Can you work these out from the model? Positions are in its coordinate system, mm. A direction names the side the tool comes from. Give positions to 0.01 mm unless a question says otherwise; leave off trailing zeros. Order: outer loops, then holes, each group sorted by start corner. A loop starts at its lowest first (then second) coordinate and runs counter-clockwise, first axis right, second up.
Item 1: If I drill on line 1 along Y through (x, z) = (-9.5, 10.5); line 2 along X through (y, z) = (38, 5); line 3 along Y through (x, z) = (14.5, -16.5), over which ranges is the centre line in solid material (lowest first)?
Item 2: I want a section at B-B, the plane y = 28.5. Write out the boundary of the cut face in (x, z).
Item 3: If we mould it in two halves opening along Z, with no side actions, what happens to faces 3 (the cylindrical face through (-10.14, 10.726, 12.559)), 4 (the cylindrical face through (-10.14, 17.16, -27.48)), 5 (the flat face through (-10, 20, -15))? For each: +Z half, -Z half, draft (parallel to the pull), parting line (faces both ways), or undercut.
Item 4: I want a section at C-C, the plane z = 22.5. Write out the boundary of the cut face in (x, y).
Item 5: I'm going to push flat-ended pins straight in: pin 1 Ø4 at (x, z) = (-5.5, 19) entering from +Y; pin 2 Ø10 at (x, z) = (5.5, -2) entering from +Y; pin 3 Ø8 at (x, z) = (0, -5.5) entering from +Y; pin 4 Ø3 at (x, z) = (-0.5, -3) entering from -Y. Where does each tip first touch, or does it pass through?
Item 6: Which directions (+Z, -Z, +X, -X, +Y, -Y) give clear straight access to the entire face, cutting with the end or side of a thin tool? Please do faces 1 (the flat face through (20, 5, 0)), 2 (the flat face through (10, 10, 0)).
Item 7: I want a section at D-D, the plane z = 5. Write out the boundary of the cut face in (x, y), then the cut area to 3 significant figures.
Item 8: I want a section at A-A, the plane x = -3.5. Write out the boundary of the cut face in (y, z), then the cut area to 3 significant figures.
```python
from build123d import *

# Parameters (mm, degrees)
SKETCH1_W              = 40
SKETCH1_H              = 61
BOSS_EXTRUDE1_DEPTH    = 40
SKETCH2_W              = 20
SKETCH2_H              = 61
CUT_EXTRUDE1_DEPTH     = 30
CUT_EXTRUDE3_START     = -20
CUT_EXTRUDE3_OUTLINE_R = 9.5
CUT_EXTRUDE3_DEPTH     = 20


# Read off the part's stored shape, not the designer's step: Cut-Extrude3
with BuildPart() as part:
    # Sketch1 → Boss-Extrude1 (new body)
    with BuildSketch(Plane(origin=(0, 0, 0), x_dir=(1, 0, 0), z_dir=(0, 1, 0))):
        Rectangle(SKETCH1_W, SKETCH1_H)
    extrude(amount=BOSS_EXTRUDE1_DEPTH)

    # Sketch2 → Cut-Extrude1 (cut)
    with BuildSketch(Plane(origin=(0, 40, 0), x_dir=(1, 0, 0), z_dir=(0, 1, 0))):
        with Locations((10, 0)):
            Rectangle(SKETCH2_W, SKETCH2_H)
    extrude(amount=-CUT_EXTRUDE1_DEPTH, mode=Mode.SUBTRACT)

    # Cut-Extrude3 outline → Cut-Extrude3 (cut)
    with BuildSketch(Plane(origin=(0, 0, 0), x_dir=(0, 0, -1), z_dir=(1, 0, 0)).offset(CUT_EXTRUDE3_START)):
        with BuildLine():
            ThreePointArc((-10.5, 40), (3.642135624, 34.142135624), (9.5, 20))
            Line((9.5, 20), (20.499888339, 20))
            ThreePointArc((20.499888339, 20), (27.554228667, 17.087755818), (30.49977668, 10.047256507))
            Line((30.49977668, 10.047256507), (30.5, 10))
            Line((30.5, 10), (30.5, 40))
            Line((30.5, 40), (-10.5, 40))
        make_face()
        with BuildLine():
            ThreePointArc((-30.5, 20), (-24.642135624, 34.142135624), (-10.5, 40))
            Line((-10.5, 40), (-30.5, 40))
            Line((-30.5, 40), (-30.5, 20))
        make_face()
        with Locations((-10.5, 20)):
            Circle(CUT_EXTRUDE3_OUTLINE_R)
    extrude(amount=CUT_EXTRUDE3_DEPTH, mode=Mode.SUBTRACT)


solid = part.part
```
Results list:
1. line 1: y = 0 to 10.5, 29.5 to 40
1. line 2: x = -20 to 0
1. line 3: y = 0 to 10
2. outline: (-20, -7.6) - (0, -7.6) - (0, 6.26) - (-20, 6.26) - close; (-20, 14.74) - (0, 14.74) - (0, 28.6) - (-20, 28.6) - close
3. face 3: undercut
3. face 4: -Z half
3. face 5: draft
4. outline: (-20, 0) - (20, 0) - (20, 10) - (0, 10) - (0, 36) - (-20, 36) - close
5. pin 1: stops at y = 38.91
5. pin 2: stops at y = 10
5. pin 3: stops at y = 36
5. pin 4: stops at y = 0
6. face 1: +Z, -Z, +X, +Y, -Y
6. face 2: +Z, -Z, +X, +Y
7. outline: (-20, 0) - (20, 0) - (20, 10) - (0, 10) - (0, 12.25) - (-20, 12.25) - close; (-20, 27.75) - (0, 27.75) - (0, 39.23) - (-20, 39.23) - close
7. area: 675 mm2
8. outline: (0, -30.5) - (10, -30.5) - (10.05, -30.5) arc R10 ccw to (20, -20.5) - (20, -9.5) arc R20 ccw to (20, 30.5) - (0, 30.5) - close; hole circle Ø19 at (20, 10.5)
8. area: 1,540 mm2
